Work out the finished part from the listing and answer in its coordinate system (mm). Face numbers are marked on the shaded views. Round coordinates to 2 decimals unless told otherwise and drop trailing zeros. Loops run counter-clockwise (first coordinate to the right, second up) from the corner with the lowest first, then second, coordinate; pieces in that order, holes last.
Autodesk Inventor part; units mm, degrees
ref_plane "YZ Plane" through (0, 0, 0) normal (1, 0, 0) x (0, 1, 0)
ref_plane "XZ Plane" through (0, 0, 0) normal (0, 1, 0) x (-1, 0, 0)
ref_plane "XY Plane" through (0, 0, 0) normal (0, 0, 1) x (1, 0, 0)
sketch "Sketch1" plane through (0, 0, 0) normal (0, 1, 0) x (-1, 0, 0)
  circle A0 centre (0, 0) radius 3.25
  circle A1 centre (0, 0) radius 2.1
  dimension "d0" = 6.5
  dimension "d1" = 4.2
extrude "Extrusion1" add sketch "Sketch1" along normal blind 7.55
sketch "Sketch2" plane through (0, 7.55, 0) normal (0, 1, 0) x (1, 0, 0)
  line L0 (0, 0) -> (0, -43.18) construction
  line L1 (-4, 0) -> (-4, -43.18)
  line L2 (4, -43.18) -> (4, 0)
  arc A0 (4, 0) -> (-4, 0) centre (0, 0) ccw
  line L3 (4, -43.18) -> (-4, -43.18)
  circle A1 centre (0, 0) radius 2.1
  point P0 (0, -21.59)
  dimension "d6" = 4
  dimension "d7" = 43.18
extrude "Extrusion2" add sketch "Sketch2" along normal blind 2
sketch "Sketch3" plane through (0, 7.55, 0) normal (0, -1, 0) x (1, 0, 0)
  circle A0 centre (0, 35.56) radius 1.5
  circle A1 centre (0, 0) radius 3.25
  dimension "d11" = 3
  dimension "d12" = 35.56
extrude "Extrusion3" cut sketch "Sketch3" against normal blind 1 contours A0
fillet "Fillet1" radius 1 2 edges at (-4, 8.55, 43.18) (4, 8.55, 43.18)
properties part number "CC-bottomHand" material "ABS Plastic"
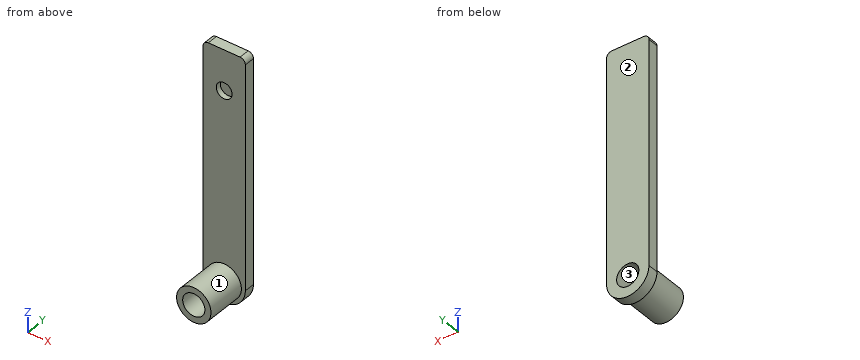
1. Given pin 1 (4 mm diameter, centred on x = 1.5, z = 21, fed in from -Y); pin 2 (2.5 mm diameter, centred on x = 0, z = 35.56, fed in from -Y); pin 3 (1 mm diameter, centred on x = 1.5, y = 6.5, fed in from -Z), each flat-ended and moving along its own axis, determine where each tip first touches the part or whether it passes through.
Answer key:
pin 1: stops at y = 7.55
pin 2: stops at y = 8.55
pin 3: stops at z = -3.09
2. Consider probe 1 along Z at (x, y) = (0, 7.75); probe 2 along Z at (x, y) = (0, 4.25); probe 3 along Y at (x, z) = (0.5, 20). Determine where each line is inside the solid, lowest interval first.
Answer key:
probe 1: z = -4 to -2.1, 2.1 to 34.06, 37.06 to 43.18
probe 2: z = -3.25 to -2.1, 2.1 to 3.25
probe 3: y = 7.55 to 9.55
3. Find section C-C (y = 7). Write down the section's boundary in (x, z).
Answer key:
outline: circle Ø6.5 at (0, 0); hole circle Ø4.2 at (0, 0)
4. Find section D-D (z = 13). Write down the section's boundary in (x, y), then the cut area to 3 significant figures.
Answer key:
outline: (-4, 7.55) - (4, 7.55) - (4, 9.55) - (-4, 9.55) - close
area: 16.0 mm2
5. Determine the mould class of the marked faces 1, 2 and 3 for opening direction Z: +Z half, -Z half, draft (parallel to the pull), parting line (faces both ways), or undercut.
Answer key:
face 1: parting line
face 2: draft
face 3: undercut
6. Find section A-A (z = 35.56). Write down the section's boundary in (x, y), then the cut area to 3 significant figures.
Answer key:
outline: (-4, 7.55) - (-1.5, 7.55) - (-1.5, 8.55) - (1.5, 8.55) - (1.5, 7.55) - (4, 7.55) - (4, 9.55) - (-4, 9.55) - close
area: 13.0 mm2
